```python
from build123d import *
from build123d import SkipClean  # not in build123d's __all__

# Parameters (mm, degrees)
F1_DEPTH  = 29.21
F3_DEPTH  = 69.05625
F5_DEPTH  = 15.4178
F7_DEPTH  = 6.9596
F9_DEPTH  = 152.4
F11_DEPTH = 89.154
F13_DEPTH = 26.4922
F15_DEPTH = 3.1496


with BuildPart() as f1:
    # F0 (on Front) → F1 (new body)
    with BuildSketch(Plane.XZ):
        with BuildLine():
            Line((11.9332703397, -4.6441399077), (17.4498, -4.6441399077))
            Line((17.4498, -4.6441399077), (17.4498, -0.8595399077))
            ThreePointArc((17.4498, -0.8595399077), (0, 16.6918600923), (-17.4498, -0.8595399077))
            Line((-17.4498, -0.8595399077), (-17.4498, -4.6441399077))
            Line((-17.4498, -4.6441399077), (-11.9332703397, -4.6441399077))
            ThreePointArc((-11.9332703397, -4.6441399077), (0, 9.1988600923), (11.9332703397, -4.6441399077))
        make_face()
    extrude(amount=F1_DEPTH)

    # F2 (on face) → F3 (join)
    with BuildSketch(Plane.XZ.offset(29.21)):
        with BuildLine():
            ThreePointArc((-9.1113708093, -4.6441399077), (0, 6.4977884545), (9.1113708093, -4.6441399077))
            Line((9.1113708093, -4.6441399077), (11.9332703397, -4.6441399077))
            ThreePointArc((11.9332703397, -4.6441399077), (0, 9.1988600923), (-11.9332703397, -4.6441399077))
            Line((-11.9332703397, -4.6441399077), (-9.1113708093, -4.6441399077))
        make_face()
        with BuildLine():
            ThreePointArc((-11.9332703397, -4.6441399077), (0, 9.1988600923), (11.9332703397, -4.6441399077))
            Line((11.9332703397, -4.6441399077), (17.4498, -4.6441399077))
            Line((17.4498, -4.6441399077), (17.4498, -0.8595399077))
            ThreePointArc((17.4498, -0.8595399077), (0, 16.6918600923), (-17.4498, -0.8595399077))
            Line((-17.4498, -0.8595399077), (-17.4498, -4.6441399077))
            Line((-17.4498, -4.6441399077), (-11.9332703397, -4.6441399077))
        make_face()
    extrude(amount=F3_DEPTH)

    # F4 (on face) → F5 (join)
    with BuildSketch(Plane.XZ.offset(98.26625)):
        with BuildLine():
            Line((15.9258256822, -4.6441399077), (15.9258256822, -0.850692377))
            ThreePointArc((15.9258256822, -0.850692377), (0, 15.1678600923), (-15.9258256822, -0.850692377))
            Line((-15.9258256822, -0.850692377), (-15.9038025792, -4.6441399077))
            Line((-15.9038025792, -4.6441399077), (-9.1113708093, -4.6441399077))
            ThreePointArc((-9.1113708093, -4.6441399077), (0, 6.4977884545), (9.1113708093, -4.6441399077))
            Line((9.1113708093, -4.6441399077), (15.9258256822, -4.6441399077))
        make_face()
    extrude(amount=F5_DEPTH)

    # F6 (on face) → F7 (join)
    with BuildSketch(Plane.XZ.offset(113.68405)):
        with BuildLine():
            ThreePointArc((-9.1113708093, -4.6441399077), (0, 6.4977884545), (9.1113708093, -4.6441399077))
            Line((9.1113708093, -4.6441399077), (15.9258256822, -4.6441399077))
            Line((15.9258256822, -4.6441399077), (15.9258256822, -0.850692377))
            ThreePointArc((15.9258256822, -0.850692377), (0, 15.1678600923), (-15.9258256822, -0.850692377))
            Line((-15.9258256822, -0.850692377), (-15.9038025792, -4.6441399077))
            Line((-15.9038025792, -4.6441399077), (-9.1113708093, -4.6441399077))
        make_face()
        with BuildLine():
            Line((15.9258256822, -0.850692377), (15.9258256822, -4.6441399077))
            Line((15.9258256822, -4.6441399077), (17.4498, -4.6441399077))
            Line((17.4498, -4.6441399077), (17.4498, -0.8595399077))
            ThreePointArc((17.4498, -0.8595399077), (0, 16.6918600923), (-17.4498, -0.8595399077))
            Line((-17.4498, -0.8595399077), (-17.4498, -4.6441399077))
            Line((-17.4498, -4.6441399077), (-15.9038025792, -4.6441399077))
            Line((-15.9038025792, -4.6441399077), (-15.9258256822, -0.850692377))
            ThreePointArc((-15.9258256822, -0.850692377), (0, 15.1678600923), (15.9258256822, -0.850692377))
        make_face()
    extrude(amount=F7_DEPTH)

    # F8 (on face) → F9 (join)
    with BuildSketch(Plane.XZ.offset(120.64365)):
        with BuildLine():
            ThreePointArc((17.4498, -0.8595399077), (0, 16.6918600923), (-17.4498, -0.8595399077))
            Line((-17.4498, -0.8595399077), (-17.4498, -4.6441399077))
            Line((-17.4498, -4.6441399077), (-9.1113708093, -4.6441399077))
            ThreePointArc((-9.1113708093, -4.6441399077), (0, 6.4977884545), (9.1113708093, -4.6441399077))
            Line((9.1113708093, -4.6441399077), (17.4498, -4.6441399077))
            Line((17.4498, -4.6441399077), (17.4498, -0.8595399077))
        make_face()
        with BuildLine():
            ThreePointArc((9.1113708093, -4.6441399077), (0, 6.4977884545), (-9.1113708093, -4.6441399077))
            Line((-9.1113708093, -4.6441399077), (-8.4364993371, -4.6441399077))
            ThreePointArc((-8.4364993371, -4.6441399077), (0, 5.8373884545), (8.4364993371, -4.6441399077))
            Line((8.4364993371, -4.6441399077), (9.1113708093, -4.6441399077))
        make_face()
    extrude(amount=F9_DEPTH)

    # F10 (on face) → F11 (join)
    with BuildSketch(Plane.XZ.offset(273.04365)):
        with BuildLine():
            ThreePointArc((17.4498, -0.8595399077), (0, 16.6918600923), (-17.4498, -0.8595399077))
            Line((-17.4498, -0.8595399077), (-17.4498, -4.6441399077))
            Line((-17.4498, -4.6441399077), (-8.4364993371, -4.6441399077))
            ThreePointArc((-8.4364993371, -4.6441399077), (0, 5.8373884545), (8.4364993371, -4.6441399077))
            Line((8.4364993371, -4.6441399077), (17.4498, -4.6441399077))
            Line((17.4498, -4.6441399077), (17.4498, -0.8595399077))
        make_face()
        with BuildLine():
            ThreePointArc((8.4364993371, -4.6441399077), (0, 5.8373884545), (-8.4364993371, -4.6441399077))
            Line((-8.4364993371, -4.6441399077), (-6.9997961445, -4.6441399077))
            ThreePointArc((-6.9997961445, -4.6441399077), (0, 4.4403884545), (6.9997961445, -4.6441399077))
            Line((6.9997961445, -4.6441399077), (8.4364993371, -4.6441399077))
        make_face()
    extrude(amount=F11_DEPTH)

    # F12 (on face) → F13 (cut)
    with BuildSketch(Plane.XZ.offset(362.19765)):
        with BuildLine():
            ThreePointArc((-16.4338, -0.8565464804), (0, 15.6758600923), (16.4338, -0.8565464805))
            Line((16.4338, -0.8565464805), (16.4338, -4.6441399077))
            Line((16.4338, -4.6441399077), (17.4498, -4.6441399077))
            Line((17.4498, -4.6441399077), (17.4498, -0.8595399077))
            ThreePointArc((17.4498, -0.8595399077), (0, 16.6918600923), (-17.4498, -0.8595399077))
            Line((-17.4498, -0.8595399077), (-17.4498, -4.6441399077))
            Line((-17.4498, -4.6441399077), (-16.4338, -4.6441399077))
            Line((-16.4338, -4.6441399077), (-16.4338, -0.8565464804))
        make_face()
    extrude(amount=-F13_DEPTH, mode=Mode.SUBTRACT)

    # F14 (on face) → F15 (join)
    with BuildSketch(Plane(origin=(0, 0, 0), x_dir=(-1, 0, 0), z_dir=(0, 1, 0))):
        with BuildLine():
            ThreePointArc((16.6878128411, -0.8551161423), (0, 15.9298600923), (-16.6878128411, -0.8551161423))
            Line((-16.6878128411, -0.8551161423), (-16.6878128411, -4.6441399077))
            Line((-16.6878128411, -4.6441399077), (-11.9332703397, -4.6441399077))
            ThreePointArc((-11.9332703397, -4.6441399077), (0, 9.1988600923), (11.9332703397, -4.6441399077))
            Line((11.9332703397, -4.6441399077), (16.6658154206, -4.6441399077))
            Line((16.6658154206, -4.6441399077), (16.6878128411, -0.8551161423))
        make_face()
    with SkipClean():  # cleaning this boolean's faces spoils the solid; the shape is the same uncleaned
        extrude(amount=F15_DEPTH)


solid = f1.part
```
CAD build for the part. Positions are in the model's coordinates, mm. A direction names the side the tool comes from. Coordinates: 2 decimals unless noted, no trailing zeros. Order: outer loops, then holes, each group sorted by start corner. A loop starts at its lowest first (then second) coordinate and runs counter-clockwise, first axis right, second up. Notation, with made-up numbers: (55, 73) - (107, 73) arc R23 cw to (107, 103) - close; hole circle Ø4 at (37, 51.25). An arc over 180 degrees is marked (long way). Answer in a Markdown table with one row per item.
1. 3-axis set-ups, long thin cutter, end or side, ignore diameter. For faces 4 (the face through (0, -113.684, 16)), 5 (the face through (-0.23, -74.287, 6.495)), 6 (the face through (-3, -335.705, 16)), 7 (the face through (0, -362.198, 6)): which of +Z, -Z, +X, -X, +Y, -Y reach the whole face in a straight line?
Answer:
| item | result |
|---|---|
| face 4 | +Z |
| face 5 | +Y |
| face 6 | +Z, -Y |
| face 7 | +Z, -Z, +X, -X, -Y |
2. Drill centre lines: L1, parallel to X at y = -241.5, z = 12; L2, parallel to Z at x = 12, y = -180.5; L3, parallel to X at y = -25.5, z = -3.25. Where is each one in solid material? Low to high. Write a range as from..to.
Answer:
| item | result |
|---|---|
| L1 | -11.91..11.91 |
| L2 | -4.64..11.91 |
| L3 | -17.45..-12.06, 12.06..17.45 |
3. Flat gauge pins, fed straight in: P1, Ø6.5, axis at x = -7, z = 1.5, coming from the +Y side; P2, Ø3, axis at y = -346.5, z = -3, coming from the -X side; P3, Ø8, axis at x = -0.5, z = 0.5, coming from the +Y side. Where does each tip first touch, or does it go through?
Answer:
| item | result |
|---|---|
| P1 | y = -29.21 |
| P2 | x = -16.43 |
| P3 | y = -273.04 |
4. Slice it at A-A, the plane x = 0. List the corners of the cut face in (y, z), then the cut area to 3 significant figures.
Answer:
| item | result |
|---|---|
| outline | (-362.2, 4.44) - (-273.04, 4.44) - (-273.04, 5.84) - (-120.64, 5.84) - (-120.64, 6.5) - (-29.21, 6.5) - (-29.21, 9.2) - (3.15, 9.2) - (3.15, 15.93) - (0, 15.93) - (0, 16.69) - (-98.27, 16.69) - (-98.27, 15.17) - (-113.68, 15.17) - (-113.68, 16.69) - (-335.71, 16.69) - (-335.71, 15.68) - (-362.2, 15.68) - close |
| area | 3,870 mm² |
5. Pull direction Y, two halves, no side cores. Call faces 1 (the face through (0.351, -105.867, 15.164)), 2 (the face through (-0.185, -316.997, 4.438)), 3 (the face through (-4, 0, 16)): +Y half, -Y half, draft (parallel to the pull), parting line (faces both ways), or undercut.
Answer:
| item | result |
|---|---|
| face 1 | undercut |
| face 2 | draft |
| face 3 | +Y half |
